Geometry check sheet. Reference: the model listing, model coordinates, mm. Face numbers are marked on the shaded views. A direction names the side the tool comes from. Give positions to 0.01 mm unless a question says otherwise; leave off trailing zeros. Loops run counter-clockwise (first coordinate to the right, second up) from the corner with the lowest first, then second, coordinate; pieces in that order, holes last. Notation, with made-up numbers: (19, 40.25) - (60, 40.25) arc R6 cw to (60, 44.25) - close; hole circle Ø11 at (-2.5, 35). An arc over 180 degrees is marked (long way). Use a Markdown table: item, result. Add a question column.
1. Set-up check for the marked faces 1, 2 and 3: record each of +Z, -Z, +X, -X, +Y, -Y from which the full face is reachable in a straight line by a thin tool's end or side.
2. Cross-section at D-D on z = -13. Enter the section's corners in (x, y).
3. Cross-section at B-B on x = 3.5. Enter the section's corners in (y, z).
4. Material ranges on L1, parallel to X at y = 1.1, z = -3; L2, parallel to Z at x = 1.5, y = 2.45; L3, parallel to Y at x = 22.5, z = -4.25, recorded low to high.
5. Cross-section at A-A on z = -19. Enter the section's corners in (x, y), and give its area (3 significant figures).
6. Depth check by flat-ended pin: P1, Ø1, axis at x = 23.5, y = 3.5, coming from the +Z side; P2, Ø1, axis at y = 3, z = -16, coming from the +X side; P3, Ø4, axis at x = 12, z = -2.5, coming from the +Y side; P4, Ø2.5, axis at x = 1.5, y = 3.5, coming from the -Z side. Enter the tip coordinate at first touch or a pass-through.
7. Cross-section at C-C on y = 1. Enter the section's corners in (x, z), and give its area (3 significant figures).
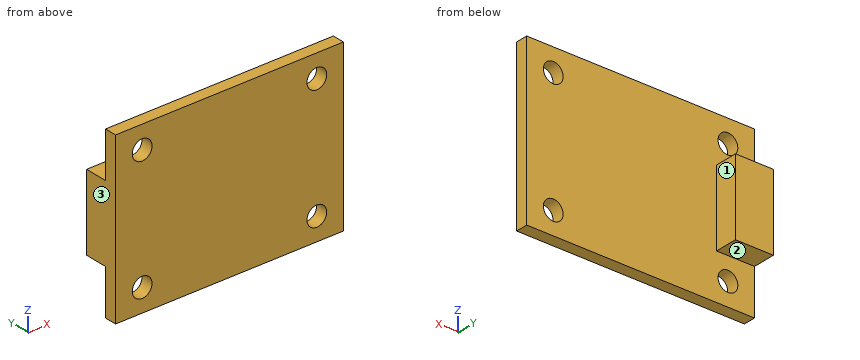
from build123d import *

# Parameters (mm, degrees)
SKETCH_1_W      = 30
SKETCH_1_H      = 22
SKETCH_1_R      = 1.3
EXTRUDE_1_DEPTH = 1.6
SKETCH_2_W      = 5
SKETCH_2_H      = 10
EXTRUDE_2_DEPTH = 3


with BuildPart() as part:
    # 草图1 → 凸台-拉伸1 (new body)
    with BuildSketch(Plane(origin=(0, 0, 0), x_dir=(1, 0, 0), z_dir=(0, 1, 0))):
        with Locations((15, 11)):
            Rectangle(SKETCH_1_W, SKETCH_1_H)
        with Locations(Location((3.5, 3, 0), (0, 0, 270))):
            Circle(SKETCH_1_R, mode=Mode.SUBTRACT)
        with Locations(Location((26.5, 3, 0), (0, 0, 270))):
            Circle(SKETCH_1_R, mode=Mode.SUBTRACT)
        with Locations(Location((26.5, 19, 0), (0, 0, 90))):
            Circle(SKETCH_1_R, mode=Mode.SUBTRACT)
        with Locations(Location((3.5, 19, 0), (0, 0, 90))):
            Circle(SKETCH_1_R, mode=Mode.SUBTRACT)
    extrude(amount=EXTRUDE_1_DEPTH)

    # 草图2 → 凸台-拉伸2 (add)
    with BuildSketch(Plane(origin=(0, 1.6, 0), x_dir=(1, 0, 0), z_dir=(0, 1, 0))):
        with Locations((2.5, 11)):
            Rectangle(SKETCH_2_W, SKETCH_2_H)
    extrude(amount=EXTRUDE_2_DEPTH)


solid = part.part
Values found:
| question | item | result |
|---|---|---|
| 1 | face 1 | +Z, -Z, +X, +Y |
| 1 | face 2 | -Z, +X, -X, +Y |
| 1 | face 3 | +Z, -Z, -X, +Y, -Y |
| 2 | outline | (0, 0) - (30, 0) - (30, 1.6) - (5, 1.6) - (5, 4.6) - (0, 4.6) - close |
| 3 | outline | (0, -22) - (1.6, -22) - (1.6, -20.3) - (0, -20.3) - close; (0, -17.7) - (1.6, -17.7) - (1.6, -16) - (4.6, -16) - (4.6, -6) - (1.6, -6) - (1.6, -4.3) - (0, -4.3) - close; (0, -1.7) - (1.6, -1.7) - (1.6, 0) - (0, 0) - close |
| 4 | L1 | x = 0 to 2.2, 4.8 to 25.2, 27.8 to 30 |
| 4 | L2 | z = -16 to -6 |
| 4 | L3 | y = 0 to 1.6 |
| 5 | outline | (0, 0) - (2.2, 0) - (2.2, 1.6) - (0, 1.6) - close; (4.8, 0) - (25.2, 0) - (25.2, 1.6) - (4.8, 1.6) - close; (27.8, 0) - (30, 0) - (30, 1.6) - (27.8, 1.6) - close |
| 5 | area | 39.7 mm2 |
| 6 | P1 | passes through |
| 6 | P2 | stops at x = 5 |
| 6 | P3 | stops at y = 1.6 |
| 6 | P4 | stops at z = -16 |
| 7 | outline | (0, -22) - (30, -22) - (30, 0) - (0, 0) - close; hole circle Ø2.6 at (3.5, -19); hole circle Ø2.6 at (3.5, -3); hole circle Ø2.6 at (26.5, -19); hole circle Ø2.6 at (26.5, -3) |
| 7 | area | 639 mm2 |
